Check sheet for the drawn part. Datum: minimum x, y, z corner. Units: mm. A direction names the side the tool comes from. Round coordinates to 2 decimals unless told otherwise and drop trailing zeros. Loops run counter-clockwise (first coordinate to the right, second up) from the corner with the lowest first, then second, coordinate; pieces in that order, holes last.
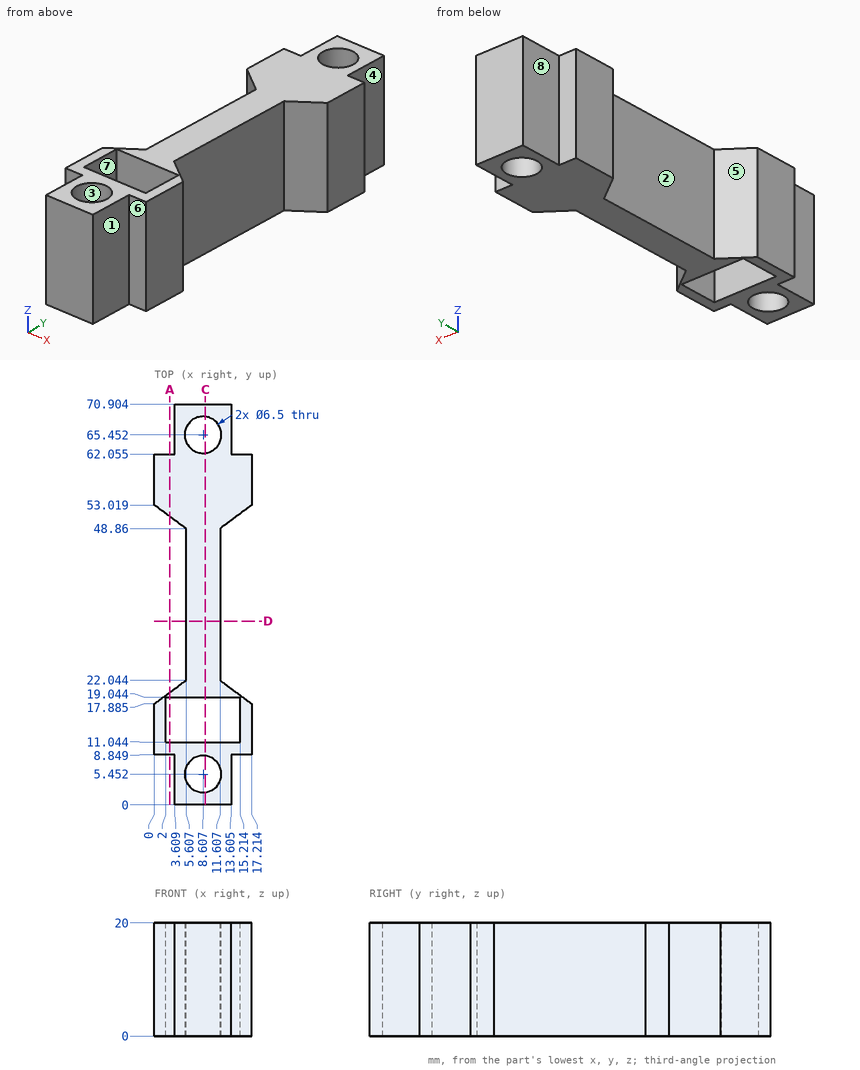
1) Sectioned sample at A-A, the plane x = 2.75. State how many separate pieces and enclosed holes the cut face has, then the cut area to 3 significant figures.
Report:
separate pieces: 3
enclosed holes: 0
area: 283 mm2
2) Sectioned sample at C-C, the plane x = 9. Record the cut outline in (y, z).
Report:
outline: (0, 0) - (2.23, 0) - (2.23, 20) - (0, 20) - close; (8.68, 0) - (11.04, 0) - (11.04, 20) - (8.68, 20) - close; (19.04, 0) - (62.23, 0) - (62.23, 20) - (19.04, 20) - close; (68.68, 0) - (70.9, 0) - (70.9, 20) - (68.68, 20) - close
3) Scan lines: line 1 along Y through (x, z) = (8.5, 17.5); line 2 along Y through (x, z) = (9.5, 17) (1 decimal); line 3 along X through (y, z) = (15.5, 14.5) (1 decimal). Record each from-to range of solid material in increasing order.
Report:
line 1: y = 0 to 2.2, 8.7 to 11.04, 19.04 to 62.2, 68.7 to 70.9
line 2: y = 0 to 2.3, 8.6 to 11, 19 to 62.3, 68.6 to 70.9
line 3: x = 0 to 2, 15.2 to 17.2
4) Sectioned sample at D-D, the plane y = 32.5. Record the cut outline in (x, z), then the cut area to 3 significant figures.
Report:
outline: (5.61, 0) - (11.61, 0) - (11.61, 20) - (5.61, 20) - close
area: 120 mm2
5) Access from +Z, -Z, +X, -X, +Y, -Y to the whole of each face (thin tool, end or side, straight path). Record for the marked faces 4, 5, 6, 7 and 8.
Report:
face 4: +Z, -Z, +X, +Y
face 5: +Z, -Z, -X
face 6: +Z, -Z, +X, -Y
face 7: +Z, -Z
face 8: +Z, -Z, -X, +Y
6) Gauge pin test, flat ends, axial feed: pin 1 (9.5 mm diameter, centred on y = 5.5, z = 14, fed in from -X); pin 2 (4.5 mm diameter, centred on y = 3.5, z = 15, fed in from +X) (1 decimal); pin 3 (1.1 mm diameter, centred on x = 1.5, z = 5.5, fed in from -Y); pin 4 (4 mm diameter, centred on y = 20.5, z = 16.5, fed in from +X) (1 decimal). Record the tip position at first contact, or that the pin passes through.
Report:
pin 1: stops at x = 0
pin 2: stops at x = 13.6
pin 3: stops at y = 8.85
pin 4: stops at x = 16.4
7) Mould release check, pull along X, two halves, no side actions. Record for the marked faces 1, 2 and 3: +X half, -X half, draft (parallel to the pull), parting line (faces both ways), or undercut.
Report:
face 1: +X half
face 2: -X half
face 3: undercut
